from build123d import *

# Parameters (mm, degrees)
SKETCH1_W           = 96
SKETCH1_H           = 86
BOSS_EXTRUDE1_DEPTH = 2
BOSS_EXTRUDE3_DEPTH = 25
SKETCH3_W           = 20
SKETCH3_H           = 30
CUT_EXTRUDE1_DEPTH  = 25
SKETCH4_W           = 14.5
SKETCH4_H           = 14.5
CUT_EXTRUDE2_DEPTH  = 25
SKETCH5_W           = 13
SKETCH5_H           = 13
CUT_EXTRUDE3_DEPTH  = 25
FILLET1_R           = 5


with BuildPart() as part:
    # Sketch1 → Boss-Extrude1 (new body)
    with BuildSketch(Plane.XY):
        with Locations((-344.5, 129.5)):
            Rectangle(SKETCH1_W, SKETCH1_H)
    extrude(amount=BOSS_EXTRUDE1_DEPTH)

    # Sketch2 → Boss-Extrude3 (add)
    with BuildSketch(Plane.XY.offset(2)):
        Polygon((-296.5, 170.5), (-296.5, 172.5), (-298.5, 172.5), (-390.5, 172.5), (-392.5, 172.5), (-392.5, 170.5), (-392.5, 86.5), (-390.5, 86.5), (-390.5, 170.5), (-298.5, 170.5), (-298.5, 86.5), (-296.5, 86.5), align=None)
    extrude(amount=BOSS_EXTRUDE3_DEPTH)

    # Sketch3 → Cut-Extrude1 (cut)
    with BuildSketch(Plane(origin=(0, 0, 0), x_dir=(-1, 0, 0), z_dir=(0, 0, -1))):
        with Locations((380.5, 155.5)):
            Rectangle(SKETCH3_W, SKETCH3_H)
    extrude(amount=-CUT_EXTRUDE1_DEPTH, mode=Mode.SUBTRACT)

    # Sketch4 → Cut-Extrude2 (cut)
    with BuildSketch(Plane(origin=(0, 0, 0), x_dir=(-1, 0, 0), z_dir=(0, 0, -1))):
        with Locations((325.75, 143.25)):
            Rectangle(SKETCH4_W, SKETCH4_H)
    extrude(amount=-CUT_EXTRUDE2_DEPTH, mode=Mode.SUBTRACT)

    # Sketch5 → Cut-Extrude3 (cut)
    with BuildSketch(Plane(origin=(0, 0, 0), x_dir=(-1, 0, 0), z_dir=(0, 0, -1))):
        with Locations((313, 111)):
            Rectangle(SKETCH5_W, SKETCH5_H)
    extrude(amount=-CUT_EXTRUDE3_DEPTH, mode=Mode.SUBTRACT)

    # Fillet1
    fillet1_edges = [part.edges().sort_by_distance(p)[0] for p in [
        (-390.5, 170.5, 13.5),
        (-298.5, 128.5, 2),
        (-298.5, 170.5, 14.5),
        (-334.5, 170.5, 2),
        (-390.5, 113.5, 2),
    ]]
    fillet(fillet1_edges, radius=FILLET1_R)


solid = part.part
Read the model definition and answer for the solid it produces. Units are mm, in the model's axes. A direction names the side the tool comes from. Give positions to 0.01 mm unless a question says otherwise; leave off trailing zeros. Loops run counter-clockwise (first coordinate to the right, second up) from the corner with the lowest first, then second, coordinate; pieces in that order, holes last. Notation, with made-up numbers: (50.25, 2) -> (99.25, 2) arc R18 ccw to (99.25, 21) -> close; hole circle Ø8 at (30.5, 25.5). An arc over 180 degrees is marked (long way). Use a Markdown table: item, result.
Q1. This flat-tipped pin is pushed along its axis until it touches: pin 1 (2 mm diameter, centred on x = -309, z = 9, fed in from -Y). Where does it stop, or does it pass through?
Solved:
| item | result |
|---|---|
| pin 1 | stops at y = 170.5 |
Q2. Section A-A, the plane y = 154.5 is taken. Determine the outline of the cut face in (x, z), then the cut area to 3 significant figures.
Solved:
| item | result |
|---|---|
| outline | (-392.5, 0) -> (-390.5, 0) -> (-390.5, 27) -> (-392.5, 27) -> close; (-370.5, 0) -> (-296.5, 0) -> (-296.5, 27) -> (-298.5, 27) -> (-298.5, 7) arc R5 cw to (-303.5, 2) -> (-370.5, 2) -> close |
| area | 257 mm^2 |
Q3. Section C-C, the plane x = -376 is taken. Determine the outline of the cut face in (y, z).
Solved:
| item | result |
|---|---|
| outline | (86.5, 0) -> (140.5, 0) -> (140.5, 2) -> (86.5, 2) -> close; (170.5, 0) -> (172.5, 0) -> (172.5, 27) -> (170.5, 27) -> close |
Q4. Section D-D, the plane z = 14.75 is taken. Determine the outline of the cut face in (x, y), then the cut area to 3 significant figures.
Solved:
| item | result |
|---|---|
| outline | (-392.5, 86.5) -> (-390.5, 86.5) -> (-390.5, 165.5) arc R5 cw to (-385.5, 170.5) -> (-303.5, 170.5) arc R5 cw to (-298.5, 165.5) -> (-298.5, 86.5) -> (-296.5, 86.5) -> (-296.5, 172.5) -> (-392.5, 172.5) -> close |
| area | 539 mm^2 |
Q5. Section B-B, the plane x = -324.5 is taken. Determine the outline of the cut face in (y, z).
Solved:
| item | result |
|---|---|
| outline | (86.5, 0) -> (136, 0) -> (136, 2) -> (86.5, 2) -> close; (150.5, 0) -> (172.5, 0) -> (172.5, 27) -> (170.5, 27) -> (170.5, 7) arc R5 cw to (165.5, 2) -> (150.5, 2) -> close |
Q6. A tool of negligible diameter and unlimited length cuts with its end or side. For faces 1 (the face through (-300, 169.07, 17.14)), 2 (the face through (-296.5, 129, 13)), 3 (the face through (-326, 136, 1)), from which of +Z, -Z, +X, -X, +Y, -Y can it reach the whole face along a straight path? Write none if from no direction.
Solved:
| item | result |
|---|---|
| face 1 | +Z, -Y |
| face 2 | +Z, -Z, +X, +Y, -Y |
| face 3 | +Z, -Z |
Q7. Find the intervals of material crossed by line 1 along X through (y, z) = (113.5, 25.5); line 2 along Y through (x, z) = (-380.5, 9.25); line 3 along Z through (x, y) = (-384, 101), in increasing order.
Solved:
| item | result |
|---|---|
| line 1 | x = -392.5 to -390.5, -298.5 to -296.5 |
| line 2 | y = 170.5 to 172.5 |
| line 3 | z = 0 to 2 |
Q8. Determine the mould class of faces 4 (the face through (-389.07, 113.88, 3.5)), 5 (the face through (-326, 150.5, 1)), 6 (the face through (-344, 172.5, 13)) for opening direction Y: pulls with the +Y half, pulls with the -Y half, needs draft (parallel to the pull), parting line crosses it, or undercut.
Solved:
| item | result |
|---|---|
| face 4 | needs draft |
| face 5 | undercut |
| face 6 | pulls with the +Y half |
